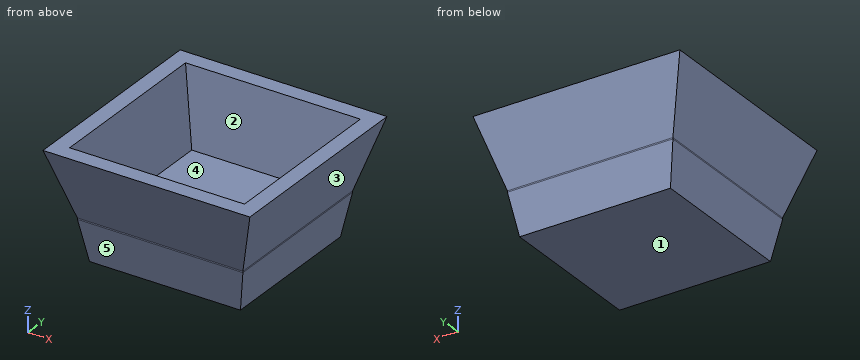
```python
from build123d import *

# Parameters (mm, degrees)
F0_W          = 19.05
F0_H          = 19.05
F0_W_2        = 12.7
F0_H_2        = 12.7
F1_DEPTH      = 6.35
F2_W          = 15.24
F2_H          = 15.24
F3_DEPTH      = 3.81
F4_SIZE2      = 6.34999
F4_SIZE       = 1.701467
F5_T4_DEPTH   = 52.0165982025
F5_T10_DEPTH  = 52.0165982025
F5_T16_DEPTH  = 52.0165982025
F5_T23_DEPTH  = 52.0165982025
F5_T29_DEPTH  = 52.0165982025
F5_T35_DEPTH  = 52.0165982025
F5_T41_DEPTH  = 52.0165982025
F5_T47_DEPTH  = 52.0165982025
F5_T54_DEPTH  = 52.0165982025
F5_T60_DEPTH  = 52.0165982025
F5_T66_DEPTH  = 52.0165982025
F5_T72_DEPTH  = 52.0165982025
F5_T78_DEPTH  = 52.0165982025
F5_T85_DEPTH  = 52.0165982025
F5_T91_DEPTH  = 52.0165982025
F5_T97_DEPTH  = 52.0165982025
F5_T103_DEPTH = 52.0165982025
F5_T109_DEPTH = 52.0165982025
F5_T116_DEPTH = 52.0165982025
F5_T122_DEPTH = 52.0165982025
F6_C1_SIZE2   = 0.6718057965
F6_C1_SIZE    = 3.81
F6_C2_SIZE2   = 0.6718057965
F6_C2_SIZE    = 3.81
F6_C3_SIZE2   = 3.81
F6_C3_SIZE    = 0.6718057965
F6_C4_SIZE2   = 3.81
F6_C4_SIZE    = 0.6718057965


# Not quite as in the source:
# - a fillet or chamfer that OpenCascade refuses, or shapes differently, is made with other operations: its cross-section is extruded or revolved along the edge and cut away or added
# - a fillet or chamfer is up to 0.001 mm smaller than in the source, because OpenCascade refuses the exact size


with BuildPart() as f1:
    # F0 (on Top) → F1 (new body)
    with BuildSketch(Plane.XY):
        Rectangle(F0_W, F0_H)
        Rectangle(F0_W_2, F0_H_2, mode=Mode.SUBTRACT)
    extrude(amount=F1_DEPTH)

    # F2 (on Top) → F3 (join)
    with BuildSketch(Plane.XY):
        Rectangle(F2_W, F2_H)
    extrude(amount=-F3_DEPTH)

    # F4 (size 1.7014773719 and 6.35 in the source; OpenCascade refuses exactly that, so slightly less here)
    f4_edges = [f1.edges().sort_by_distance(p)[0] for p in [
        (0, 6.35, 6.35),
        (6.35, 0, 6.35),
        (0, -6.35, 6.35),
        (-6.35, 0, 6.35),
    ]]
    f4_side = f1.faces().sort_by_distance((9.255592, 0, 6.35))[0]
    chamfer(f4_edges, length=F4_SIZE, length2=F4_SIZE2, reference=f4_side)

    # F5: chamfer of 6.35 x 1.9413898273 on 4 edges, made by hand


with BuildPart() as f5_tool2:
    # F5_s3 → F5_t4 (new body)
    with BuildSketch(Plane.YZ.offset(26.0082991012)):
        Polygon((9.525, 6.35), (7.5836101727, 0), (9.525, 0), align=None)
    extrude(amount=-F5_T4_DEPTH)

    split(bisect_by=Plane.XZ.offset(-7.62), keep=Keep.BOTTOM)

    split(bisect_by=Plane.YZ.offset(7.62), keep=Keep.TOP)


with BuildPart() as f1_1:
    add(f1.part)

    # F5_t1: cut F5_tool2
    add(f5_tool2.part, mode=Mode.SUBTRACT)


with BuildPart() as f5_tool8:
    # F5_s9 → F5_t10 (new body)
    with BuildSketch(Plane.YZ.offset(26.0082991012)):
        Polygon((9.525, 6.35), (7.5836101727, 0), (9.525, 0), align=None)
    extrude(amount=-F5_T10_DEPTH)

    split(bisect_by=Plane.XZ.offset(-7.62), keep=Keep.TOP)

    split(bisect_by=Plane.YZ.offset(7.62), keep=Keep.TOP)


with BuildPart() as f1_2:
    add(f1_1.part)

    # F5_t7: cut F5_tool8
    add(f5_tool8.part, mode=Mode.SUBTRACT)


with BuildPart() as f5_tool14:
    # F5_s15 → F5_t16 (new body)
    with BuildSketch(Plane.YZ.offset(26.0082991012)):
        Polygon((9.525, 6.35), (7.5836101727, 0), (9.525, 0), align=None)
    extrude(amount=-F5_T16_DEPTH)

    split(bisect_by=Plane.XZ.offset(-7.62), keep=Keep.BOTTOM)

    split(bisect_by=Plane.YZ.offset(-7.62), keep=Keep.TOP)

    split(bisect_by=Plane.YZ.offset(7.62), keep=Keep.BOTTOM)


with BuildPart() as f1_3:
    add(f1_2.part)

    # F5_t13: cut F5_tool14
    add(f5_tool14.part, mode=Mode.SUBTRACT)


with BuildPart() as f5_tool21:
    # F5_s22 → F5_t23 (new body)
    with BuildSketch(Plane.YZ.offset(26.0082991012)):
        Polygon((9.525, 6.35), (7.5836101727, 0), (9.525, 0), align=None)
    extrude(amount=-F5_T23_DEPTH)

    split(bisect_by=Plane.XZ.offset(-7.62), keep=Keep.BOTTOM)

    split(bisect_by=Plane.YZ.offset(-7.62), keep=Keep.BOTTOM)


with BuildPart() as f1_4:
    add(f1_3.part)

    # F5_t20: cut F5_tool21
    add(f5_tool21.part, mode=Mode.SUBTRACT)


with BuildPart() as f5_tool27:
    # F5_s28 → F5_t29 (new body)
    with BuildSketch(Plane.YZ.offset(26.0082991012)):
        Polygon((9.525, 6.35), (7.5836101727, 0), (9.525, 0), align=None)
    extrude(amount=-F5_T29_DEPTH)

    split(bisect_by=Plane.XZ.offset(-7.62), keep=Keep.TOP)

    split(bisect_by=Plane.YZ.offset(-7.62), keep=Keep.BOTTOM)


with BuildPart() as f1_5:
    add(f1_4.part)

    # F5_t26: cut F5_tool27
    add(f5_tool27.part, mode=Mode.SUBTRACT)


with BuildPart() as f5_tool33:
    # F5_s34 → F5_t35 (new body)
    with BuildSketch(Plane.XZ.offset(26.0082991012)):
        Polygon((9.525, 6.35), (7.5836101727, 0), (9.525, 0), align=None)
    extrude(amount=-F5_T35_DEPTH)

    split(bisect_by=Plane.XZ.offset(7.62), keep=Keep.TOP)

    split(bisect_by=Plane.YZ.offset(7.62), keep=Keep.TOP)


with BuildPart() as f1_6:
    add(f1_5.part)

    # F5_t32: cut F5_tool33
    add(f5_tool33.part, mode=Mode.SUBTRACT)


with BuildPart() as f5_tool39:
    # F5_s40 → F5_t41 (new body)
    with BuildSketch(Plane.XZ.offset(26.0082991012)):
        Polygon((9.525, 6.35), (7.5836101727, 0), (9.525, 0), align=None)
    extrude(amount=-F5_T41_DEPTH)

    split(bisect_by=Plane.XZ.offset(7.62), keep=Keep.TOP)

    split(bisect_by=Plane.YZ.offset(7.62), keep=Keep.BOTTOM)


with BuildPart() as f1_7:
    add(f1_6.part)

    # F5_t38: cut F5_tool39
    add(f5_tool39.part, mode=Mode.SUBTRACT)


with BuildPart() as f5_tool45:
    # F5_s46 → F5_t47 (new body)
    with BuildSketch(Plane.XZ.offset(26.0082991012)):
        Polygon((9.525, 6.35), (7.5836101727, 0), (9.525, 0), align=None)
    extrude(amount=-F5_T47_DEPTH)

    split(bisect_by=Plane.XZ.offset(-7.62), keep=Keep.TOP)

    split(bisect_by=Plane.XZ.offset(7.62), keep=Keep.BOTTOM)

    split(bisect_by=Plane.YZ.offset(7.62), keep=Keep.TOP)


with BuildPart() as f1_8:
    add(f1_7.part)

    # F5_t44: cut F5_tool45
    add(f5_tool45.part, mode=Mode.SUBTRACT)


with BuildPart() as f5_tool52:
    # F5_s53 → F5_t54 (new body)
    with BuildSketch(Plane.XZ.offset(26.0082991012)):
        Polygon((9.525, 6.35), (7.5836101727, 0), (9.525, 0), align=None)
    extrude(amount=-F5_T54_DEPTH)

    split(bisect_by=Plane.XZ.offset(-7.62), keep=Keep.BOTTOM)

    split(bisect_by=Plane.YZ.offset(7.62), keep=Keep.TOP)


with BuildPart() as f1_9:
    add(f1_8.part)

    # F5_t51: cut F5_tool52
    add(f5_tool52.part, mode=Mode.SUBTRACT)


with BuildPart() as f5_tool58:
    # F5_s59 → F5_t60 (new body)
    with BuildSketch(Plane.XZ.offset(26.0082991012)):
        Polygon((9.525, 6.35), (7.5836101727, 0), (9.525, 0), align=None)
    extrude(amount=-F5_T60_DEPTH)

    split(bisect_by=Plane.XZ.offset(-7.62), keep=Keep.BOTTOM)

    split(bisect_by=Plane.YZ.offset(7.62), keep=Keep.BOTTOM)


with BuildPart() as f1_10:
    add(f1_9.part)

    # F5_t57: cut F5_tool58
    add(f5_tool58.part, mode=Mode.SUBTRACT)


with BuildPart() as f5_tool64:
    # F5_s65 → F5_t66 (new body)
    with BuildSketch(Plane.YZ.offset(-26.0082991012)):
        Polygon((-9.525, 6.35), (-7.5836101727, 0), (-9.525, 0), align=None)
    extrude(amount=F5_T66_DEPTH)

    split(bisect_by=Plane.YZ.offset(-7.62), keep=Keep.BOTTOM)

    split(bisect_by=Plane.XZ.offset(7.62), keep=Keep.TOP)


with BuildPart() as f1_11:
    add(f1_10.part)

    # F5_t63: cut F5_tool64
    add(f5_tool64.part, mode=Mode.SUBTRACT)


with BuildPart() as f5_tool70:
    # F5_s71 → F5_t72 (new body)
    with BuildSketch(Plane.YZ.offset(-26.0082991012)):
        Polygon((-9.525, 6.35), (-7.5836101727, 0), (-9.525, 0), align=None)
    extrude(amount=F5_T72_DEPTH)

    split(bisect_by=Plane.YZ.offset(-7.62), keep=Keep.BOTTOM)

    split(bisect_by=Plane.XZ.offset(7.62), keep=Keep.BOTTOM)


with BuildPart() as f1_12:
    add(f1_11.part)

    # F5_t69: cut F5_tool70
    add(f5_tool70.part, mode=Mode.SUBTRACT)


with BuildPart() as f5_tool76:
    # F5_s77 → F5_t78 (new body)
    with BuildSketch(Plane.YZ.offset(-26.0082991012)):
        Polygon((-9.525, 6.35), (-7.5836101727, 0), (-9.525, 0), align=None)
    extrude(amount=F5_T78_DEPTH)

    split(bisect_by=Plane.YZ.offset(-7.62), keep=Keep.TOP)

    split(bisect_by=Plane.XZ.offset(7.62), keep=Keep.TOP)

    split(bisect_by=Plane.YZ.offset(7.62), keep=Keep.BOTTOM)


with BuildPart() as f1_13:
    add(f1_12.part)

    # F5_t75: cut F5_tool76
    add(f5_tool76.part, mode=Mode.SUBTRACT)


with BuildPart() as f5_tool83:
    # F5_s84 → F5_t85 (new body)
    with BuildSketch(Plane.YZ.offset(-26.0082991012)):
        Polygon((-9.525, 6.35), (-7.5836101727, 0), (-9.525, 0), align=None)
    extrude(amount=F5_T85_DEPTH)

    split(bisect_by=Plane.XZ.offset(7.62), keep=Keep.TOP)

    split(bisect_by=Plane.YZ.offset(7.62), keep=Keep.TOP)


with BuildPart() as f1_14:
    add(f1_13.part)

    # F5_t82: cut F5_tool83
    add(f5_tool83.part, mode=Mode.SUBTRACT)


with BuildPart() as f5_tool89:
    # F5_s90 → F5_t91 (new body)
    with BuildSketch(Plane.YZ.offset(-26.0082991012)):
        Polygon((-9.525, 6.35), (-7.5836101727, 0), (-9.525, 0), align=None)
    extrude(amount=F5_T91_DEPTH)

    split(bisect_by=Plane.XZ.offset(7.62), keep=Keep.BOTTOM)

    split(bisect_by=Plane.YZ.offset(7.62), keep=Keep.TOP)


with BuildPart() as f1_15:
    add(f1_14.part)

    # F5_t88: cut F5_tool89
    add(f5_tool89.part, mode=Mode.SUBTRACT)


with BuildPart() as f5_tool95:
    # F5_s96 → F5_t97 (new body)
    with BuildSketch(Plane.XZ.offset(-26.0082991012)):
        Polygon((-9.525, 6.35), (-7.5836101727, 0), (-9.525, 0), align=None)
    extrude(amount=F5_T97_DEPTH)

    split(bisect_by=Plane.XZ.offset(-7.62), keep=Keep.BOTTOM)

    split(bisect_by=Plane.YZ.offset(-7.62), keep=Keep.BOTTOM)


with BuildPart() as f1_16:
    add(f1_15.part)

    # F5_t94: cut F5_tool95
    add(f5_tool95.part, mode=Mode.SUBTRACT)


with BuildPart() as f5_tool101:
    # F5_s102 → F5_t103 (new body)
    with BuildSketch(Plane.XZ.offset(-26.0082991012)):
        Polygon((-9.525, 6.35), (-7.5836101727, 0), (-9.525, 0), align=None)
    extrude(amount=F5_T103_DEPTH)

    split(bisect_by=Plane.XZ.offset(-7.62), keep=Keep.BOTTOM)

    split(bisect_by=Plane.YZ.offset(-7.62), keep=Keep.TOP)


with BuildPart() as f1_17:
    add(f1_16.part)

    # F5_t100: cut F5_tool101
    add(f5_tool101.part, mode=Mode.SUBTRACT)


with BuildPart() as f5_tool107:
    # F5_s108 → F5_t109 (new body)
    with BuildSketch(Plane.XZ.offset(-26.0082991012)):
        Polygon((-9.525, 6.35), (-7.5836101727, 0), (-9.525, 0), align=None)
    extrude(amount=F5_T109_DEPTH)

    split(bisect_by=Plane.XZ.offset(-7.62), keep=Keep.TOP)

    split(bisect_by=Plane.YZ.offset(-7.62), keep=Keep.BOTTOM)

    split(bisect_by=Plane.XZ.offset(7.62), keep=Keep.BOTTOM)


with BuildPart() as f1_18:
    add(f1_17.part)

    # F5_t106: cut F5_tool107
    add(f5_tool107.part, mode=Mode.SUBTRACT)


with BuildPart() as f5_tool114:
    # F5_s115 → F5_t116 (new body)
    with BuildSketch(Plane.XZ.offset(-26.0082991012)):
        Polygon((-9.525, 6.35), (-7.5836101727, 0), (-9.525, 0), align=None)
    extrude(amount=F5_T116_DEPTH)

    split(bisect_by=Plane.YZ.offset(-7.62), keep=Keep.BOTTOM)

    split(bisect_by=Plane.XZ.offset(7.62), keep=Keep.TOP)


with BuildPart() as f1_19:
    add(f1_18.part)

    # F5_t113: cut F5_tool114
    add(f5_tool114.part, mode=Mode.SUBTRACT)


with BuildPart() as f5_tool120:
    # F5_s121 → F5_t122 (new body)
    with BuildSketch(Plane.XZ.offset(-26.0082991012)):
        Polygon((-9.525, 6.35), (-7.5836101727, 0), (-9.525, 0), align=None)
    extrude(amount=F5_T122_DEPTH)

    split(bisect_by=Plane.YZ.offset(-7.62), keep=Keep.TOP)

    split(bisect_by=Plane.XZ.offset(7.62), keep=Keep.TOP)


with BuildPart() as f1_20:
    add(f1_19.part)

    # F5_t119: cut F5_tool120
    add(f5_tool120.part, mode=Mode.SUBTRACT)

    # F6: chamfer of 3.81 x 0.6718057965 on 4 edges, made by hand

    # F6_c1
    f6_c1_edges = [f1_20.edges().sort_by_distance(p)[0] for p in [
        (0, -7.62, -3.81),
    ]]
    f6_c1_side = f1_20.faces().sort_by_distance((0, -7.62, -3.7965638841))[0]
    chamfer(f6_c1_edges, length=F6_C1_SIZE, length2=F6_C1_SIZE2, reference=f6_c1_side)

    # F6_c2
    f6_c2_edges = [f1_20.edges().sort_by_distance(p)[0] for p in [
        (7.62, 0.3359028982, -3.81),
    ]]
    f6_c2_side = f1_20.faces().sort_by_distance((7.62, 0.3359028982, -3.7965638841))[0]
    chamfer(f6_c2_edges, length=F6_C2_SIZE, length2=F6_C2_SIZE2, reference=f6_c2_side)

    # F6_c3
    f6_c3_edges = [f1_20.edges().sort_by_distance(p)[0] for p in [
        (-0.3359028982, 7.62, -3.81),
    ]]
    f6_c3_side = f1_20.faces().sort_by_distance((-0.3359028982, 7.6065638841, -3.81))[0]
    chamfer(f6_c3_edges, length=F6_C3_SIZE, length2=F6_C3_SIZE2, reference=f6_c3_side)

    # F6_c4
    f6_c4_edges = [f1_20.edges().sort_by_distance(p)[0] for p in [
        (-7.62, 0, -3.81),
    ]]
    f6_c4_side = f1_20.faces().sort_by_distance((-7.6065638841, 0, -3.81))[0]
    chamfer(f6_c4_edges, length=F6_C4_SIZE, length2=F6_C4_SIZE2, reference=f6_c4_side)


solid = f1_20.part
```
Verification items for the finished model (mm, model axes). Face numbers are marked on the shaded views. A direction names the side the tool comes from. Coordinates: 2 decimals unless noted, no trailing zeros. Loops run counter-clockwise (first coordinate to the right, second up) from the corner with the lowest first, then second, coordinate; pieces in that order, holes last. Notation, with made-up numbers: (34, -14) -> (59, -14) arc R26 ccw to (59, 7) -> close; hole circle Ø7 at (1.5, 87.25). An arc over 180 degrees is marked (long way). Answer in a Markdown table with one row per item. Add a question column.
1. Draft check along X on the marked faces 3, 4 and 5. Enter one of: +X half, -X half, draft (parallel to the pull), parting line (faces both ways), or undercut.
2. Access from +Z, -Z, +X, -X, +Y, -Y to the whole of each face (thin tool, end or side, straight path). Record for the marked faces 1 and 2.
3. Depth check by flat-ended pin: P1, Ø1.5, axis at y = 1, z = 4, coming from the +X side; P2, Ø3, axis at x = 2, z = -2.5, coming from the +Y side; P3, Ø4, axis at x = -5.5, z = 3.5, coming from the -Y side. Enter the tip coordinate at first touch or a pass-through.
4. Section check C-C, the plane z = 3. Enter the section's corners in (x, y), then the cut area to 3 significant figures.
5. Material ranges on probe 1 along Z at (x, y) = (-4.5, 0); probe 2 along X at (y, z) = (5.75, 3); probe 3 along Y at (x, z) = (6.5, 3.5), recorded low to high. Write a range as [from, to].
6. Section check D-D, the plane z = 5.75. Enter the section's corners in (x, y), then the cut area to 3 significant figures.
Derived:
| question | item | result |
|---|---|---|
| 1 | face 3 | +X half |
| 1 | face 4 | undercut |
| 1 | face 5 | draft |
| 2 | face 1 | -Z, +X, -X, +Y, -Y |
| 2 | face 2 | +Z |
| 3 | P1 | stops at x = 9.04 |
| 3 | P2 | stops at y = 7.44 |
| 3 | P3 | stops at y = -9.27 |
| 4 | outline | (-8.5, -8.5) -> (8.5, -8.5) -> (8.5, 8.5) -> (-8.5, 8.5) -> close; hole (-7.15, -7.15) -> (7.15, -7.15) -> (7.15, 7.15) -> (-7.15, 7.15) -> close |
| 4 | area | 84.3 mm² |
| 5 | probe 1 | z = [-3.81, 0] |
| 5 | probe 2 | x = [-8.5, -7.15], [7.15, 8.5] |
| 5 | probe 3 | y = [-8.65, -7.29], [7.29, 8.65] |
| 6 | outline | (-9.34, -9.34) -> (9.34, -9.34) -> (9.34, 9.34) -> (-9.34, 9.34) -> close; hole (-7.89, -7.89) -> (7.89, -7.89) -> (7.89, 7.89) -> (-7.89, 7.89) -> close |
| 6 | area | 100 mm² |
